```python
from build123d import *

# Parameters (mm, degrees)
F1_DEPTH       = 6.35
F2_R           = 3.81
F3_DEPTH       = 6.35
F5_D           = 2.032
F5_CSINK_D     = 3.175
F5_CSINK_ANGLE = 82
F6_D           = 2.032
F6_CSINK_D     = 3.175
F6_CSINK_ANGLE = 82


with BuildPart() as f1:
    # F0 (on Top) → F1 (new body)
    with BuildSketch(Plane.XY):
        with BuildLine():
            ThreePointArc((-5.08, 12.7), (-3.5921024484, 9.1078975516), (0, 7.62))
            Line((0, 7.62), (0, 12.7))
            Line((0, 12.7), (0, 17.78))
            ThreePointArc((0, 17.78), (-3.5921024484, 16.2921024484), (-5.08, 12.7))
        make_face()
        with BuildLine():
            Line((0, 12.7), (0, 7.62))
            ThreePointArc((0, 7.62), (3.5921024484, 9.1078975516), (5.08, 12.7))
            ThreePointArc((5.08, 12.7), (3.5921024484, 16.2921024484), (0, 17.78))
            Line((0, 17.78), (0, 12.7))
        make_face()
        with BuildLine():
            ThreePointArc((5.08, 12.7), (3.5921024484, 9.1078975516), (0, 7.62))
            ThreePointArc((0, 7.62), (-3.5921024484, 9.1078975516), (-5.08, 12.7))
            Line((-5.08, 12.7), (-5.08, 0))
            ThreePointArc((-5.08, 0), (0, -5.08), (5.08, 0))
            Line((5.08, 0), (5.08, 12.7))
        make_face()
        with BuildLine():
            ThreePointArc((0, 17.78), (3.5921024484, 16.2921024484), (5.08, 12.7))
            Line((5.08, 12.7), (5.08, 32.7368881382))
            Line((5.08, 32.7368881382), (4.2115108686, 31.4493000504))
            ThreePointArc((4.2115108686, 31.4493000504), (2.384915539, 29.8046262283), (0, 29.21))
            Line((0, 29.21), (0, 17.78))
        make_face()
        with BuildLine():
            Line((-5.08, 34.29), (-5.08, 12.7))
            ThreePointArc((-5.08, 12.7), (-3.5921024484, 16.2921024484), (0, 17.78))
            Line((0, 17.78), (0, 29.21))
            ThreePointArc((0, 29.21), (-3.5921024484, 30.6978975516), (-5.08, 34.29))
        make_face()
        with BuildLine():
            Line((5.08, 34.29), (5.08, 32.7368881382))
            Line((5.08, 32.7368881382), (7.5087984569, 36.3377299308))
            Line((7.5087984569, 36.3377299308), (9.9375969139, 39.9385717235))
            Line((9.9375969139, 39.9385717235), (12.3663953708, 43.5394135161))
            Line((12.3663953708, 43.5394135161), (14.7951938277, 47.1402553087))
            Line((14.7951938277, 47.1402553087), (15.5743106671, 48.2953435247))
            Line((15.5743106671, 48.2953435247), (17.2219166379, 50.7380198285))
            Line((17.2219166379, 50.7380198285), (19.6507150948, 54.3388616211))
            Line((19.6507150948, 54.3388616211), (22.0795135518, 57.9397034137))
            Line((22.0795135518, 57.9397034137), (24.5083120087, 61.5405452064))
            Line((24.5083120087, 61.5405452064), (26.9371104656, 65.141386999))
            ThreePointArc((26.9371104656, 65.141386999), (25.5662995467, 72.1935978172), (18.5140887285, 70.8227868983))
            Line((18.5140887285, 70.8227868983), (-4.2115108686, 37.1306999496))
            ThreePointArc((-4.2115108686, 37.1306999496), (-0.9693096965, 39.2766660919), (2.8406999496, 38.5015108686))
            ThreePointArc((2.8406999496, 38.5015108686), (4.4853737717, 36.674915539), (5.08, 34.29))
        make_face()
        with BuildLine():
            Line((4.2115108686, 31.4493000504), (5.08, 32.7368881382))
            Line((5.08, 32.7368881382), (5.08, 34.29))
            ThreePointArc((5.08, 34.29), (4.4853737717, 36.674915539), (2.8406999496, 38.5015108686))
            Line((2.8406999496, 38.5015108686), (0, 34.29))
            Line((0, 34.29), (0, 29.21))
            ThreePointArc((0, 29.21), (2.384915539, 29.8046262283), (4.2115108686, 31.4493000504))
        make_face()
        Polygon((7.5087984569, 36.3377299308), (5.08, 32.7368881382), (11.5576660786, 30.9871907177), align=None)
        with BuildLine():
            ThreePointArc((-4.2115108686, 37.1306999496), (-4.8580281603, 35.77524826), (-5.08, 34.29))
            ThreePointArc((-5.08, 34.29), (-3.5921024484, 30.6978975516), (0, 29.21))
            Line((0, 29.21), (0, 34.29))
            Line((0, 34.29), (2.8406999496, 38.5015108686))
            ThreePointArc((2.8406999496, 38.5015108686), (-0.9693096965, 39.2766660919), (-4.2115108686, 37.1306999496))
        make_face()
        Polygon((9.9375969139, 39.9385717235), (7.5087984569, 36.3377299308), (13.9886397713, 34.5961055653), align=None)
        Polygon((12.3663953708, 43.5394135161), (9.9375969139, 39.9385717235), (16.4107760502, 38.1919007837), align=None)
        Polygon((14.7951938277, 47.1402553087), (12.3663953708, 43.5394135161), (18.842780956, 41.8023465243), align=None)
        Polygon((30.9680322355, 59.8029524158), (26.9371104656, 65.141386999), (24.5083120087, 61.5405452064), align=None)
        Polygon((15.5743106671, 48.2953435247), (14.7951938277, 47.1402553087), (21.262849157, 45.3950715667), (17.2219166379, 50.7380198285), align=None)
        Polygon((28.5414772497, 56.2005973827), (24.5083120087, 61.5405452064), (22.0795135518, 57.9397034137), align=None)
        Polygon((26.1149222639, 52.5982423497), (22.0795135518, 57.9397034137), (19.6507150948, 54.3388616211), align=None)
        Polygon((19.6507150948, 54.3388616211), (17.2219166379, 50.7380198285), (23.6883672781, 48.9958873167), align=None)
    extrude(amount=F1_DEPTH)

    # F2 (on face) → F3 (join)
    with BuildSketch(Plane.XY.offset(6.35)):
        with Locations((0, 12.7)):
            Circle(F2_R)
    extrude(amount=F3_DEPTH)

    # F5 (through all)
    with Locations(Plane.XY.offset(12.7)):
        with Locations((0, 12.7)):
            CounterSinkHole(F5_D / 2, F5_CSINK_D / 2, counter_sink_angle=F5_CSINK_ANGLE)

    # F6 (through all)
    with Locations(Plane(origin=(0, 0, 0), x_dir=(1, 0, 0), z_dir=(0, 0, -1))):
        with Locations((0, 0)):
            CounterSinkHole(F6_D / 2, F6_CSINK_D / 2, counter_sink_angle=F6_CSINK_ANGLE)


solid = f1.part
```
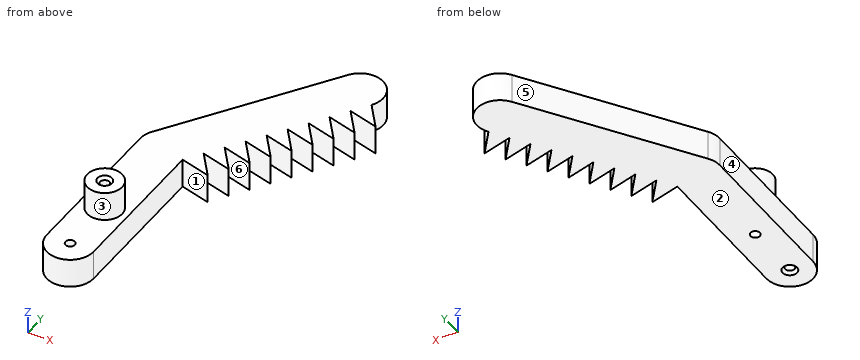
Verification items for the finished model (mm, model axes). Face numbers are marked on the shaded views. A direction names the side the tool comes from. Coordinates: 2 decimals unless noted, no trailing zeros. Loops run counter-clockwise (first coordinate to the right, second up) from the corner with the lowest first, then second, coordinate; pieces in that order, holes last. Notation, with made-up numbers: (73, 21.5) -> (125, 21.5) arc R15 cw to (125, 48.5) -> close; hole circle Ø7 at (55, 5.5). An arc over 180 degrees is marked (long way). Answer in a Markdown table with one row per item. Add a question column.
1. Section check C-C, the plane z = 9.5. Enter the section's corners in (x, y).
2. Section check D-D, the plane y = 4. Enter the section's corners in (x, z), then the cut area to 3 significant figures.
3. Depth check by flat-ended pin: P1, Ø1, axis at x = 20.5, y = 46, coming from the +Z side; P2, Ø2.5, axis at x = 0, y = 0, coming from the -Z side; P3, Ø1, axis at y = 33, z = 3.5, coming from the +X side. Enter the tip coordinate at first touch or a pass-through.
4. Section check A-A, the plane y = 12.7. Enter the section's corners in (x, z), then the cut area to 3 significant figures.
5. Material ranges on probe 1 along Y at (x, z) = (0, 7.75); probe 2 along X at (y, z) = (12.7, 3.5); probe 3 along Y at (x, z) = (15, 3.5) (3 decimals), recorded low to high. Write a range as [from, to].
6. Access from +Z, -Z, +X, -X, +Y, -Y to the whole of each face (thin tool, end or side, straight path). Record for the marked faces 1, 2 and 3.
7. Draft check along Y on the marked faces 4, 5 and 6. Enter one of: +Y half, -Y half, draft (parallel to the pull), parting line (faces both ways), or undercut.
8. Section check B-B, the plane x = 0. Enter the section's corners in (y, z), then the cut area to 3 significant figures.
Derived:
| question | item | result |
|---|---|---|
| 1 | outline | circle Ø7.62 at (0, 12.7); hole circle Ø2.03 at (0, 12.7) |
| 2 | outline | (-5.08, 0) -> (5.08, 0) -> (5.08, 6.35) -> (-5.08, 6.35) -> close |
| 2 | area | 64.5 mm² |
| 3 | P1 | stops at z = 6.35 |
| 3 | P2 | stops at z = 0.39 |
| 3 | P3 | stops at x = 10.41 |
| 4 | outline | (-5.08, 0) -> (-1.02, 0) -> (-1.02, 12.04) -> (-1.59, 12.7) -> (-3.81, 12.7) -> (-3.81, 6.35) -> (-5.08, 6.35) -> close; (1.02, 0) -> (5.08, 0) -> (5.08, 6.35) -> (3.81, 6.35) -> (3.81, 12.7) -> (1.59, 12.7) -> (1.02, 12.04) -> close |
| 4 | area | 86.7 mm² |
| 5 | probe 1 | y = [8.89, 11.68], [13.72, 16.51] |
| 5 | probe 2 | x = [-5.08, -1.02], [1.02, 5.08] |
| 5 | probe 3 | y = [38.573, 40.057], [42.833, 46.87], [47.085, 65.613] |
| 6 | face 1 | +Z, -Z, -Y |
| 6 | face 2 | -Z, +X, -X, +Y, -Y |
| 6 | face 3 | +Z |
| 7 | face 4 | draft |
| 7 | face 5 | +Y half |
| 7 | face 6 | undercut |
| 8 | outline | (-5.08, 0) -> (-1.59, 0) -> (-1.02, 0.66) -> (-1.02, 6.35) -> (-5.08, 6.35) -> close; (1.02, 0.66) -> (1.59, 0) -> (11.68, 0) -> (11.68, 12.04) -> (11.11, 12.7) -> (8.89, 12.7) -> (8.89, 6.35) -> (1.02, 6.35) -> close; (13.72, 0) -> (43.37, 0) -> (43.37, 6.35) -> (16.51, 6.35) -> (16.51, 12.7) -> (14.29, 12.7) -> (13.72, 12.04) -> close |
| 8 | area | 317 mm² |
